The listing builds one solid part. Answer for the finished solid, in the listing's coordinates (mm). Give positions to 0.01 mm unless a question says otherwise; leave off trailing zeros. Order: outer loops, then holes, each group sorted by start corner. A loop starts at its lowest first (then second) coordinate and runs counter-clockwise, first axis right, second up. Notation, with made-up numbers: (86, 41) -> (131, 41) arc R9 ccw to (131, 47) -> close; hole circle Ø4 at (-14.5, 4). An arc over 180 degrees is marked (long way). Write item = value, one per line. Start each with the question number.
```python
from build123d import *

# Parameters (mm, degrees)
BOSS_EXTRUDE1_DEPTH = 5.08
SKETCH5_W           = 7.112
SKETCH5_H           = 7.112
SKETCH5_W_2         = 2.794
SKETCH5_H_2         = 43.434
CUT_EXTRUDE1_DEPTH  = 6.08


with BuildPart() as part:
    # Sketch1 → Boss-Extrude1 (new body)
    with BuildSketch(Plane.XY):
        Polygon((-4.120444444, 6.35), (53.34, 6.35), (53.34, -95.25), (16.22499019, -95.25), (-16.356614113, -78.274710363), (-26.416, -57.15), align=None)
    extrude(amount=BOSS_EXTRUDE1_DEPTH)

    # Sketch5 → Cut-Extrude1 (cut, through all)
    with BuildSketch(Plane(origin=(0, 0, 0), x_dir=(-1, 0, 0), z_dir=(0, 0, -1))):
        with Locations((-36.83, -17.78)):
            Rectangle(SKETCH5_W, SKETCH5_H)
        with Locations((-39.37, -45.72)):
            Rectangle(SKETCH5_W, SKETCH5_H)
        with Locations((-36.83, -27.94)):
            Rectangle(SKETCH5_W, SKETCH5_H)
        with Locations((-41.91, -64.77)):
            Rectangle(SKETCH5_W, SKETCH5_H)
        with Locations((-41.91, -83.82)):
            Rectangle(SKETCH5_W, SKETCH5_H)
        with Locations((-22.098, -17.78)):
            Rectangle(SKETCH5_W, SKETCH5_H)
        with Locations((-22.098, -27.94)):
            Rectangle(SKETCH5_W, SKETCH5_H)
        with Locations((-23.622, -45.72)):
            Rectangle(SKETCH5_W, SKETCH5_H)
        with Locations((-25.146, -64.77)):
            Rectangle(SKETCH5_W, SKETCH5_H)
        with Locations((-15.367, -26.543)):
            Rectangle(SKETCH5_W_2, SKETCH5_H_2)
        with Locations((-0.127, -26.543)):
            Rectangle(SKETCH5_W_2, SKETCH5_H_2)
    extrude(amount=-CUT_EXTRUDE1_DEPTH, mode=Mode.SUBTRACT)


solid = part.part
```
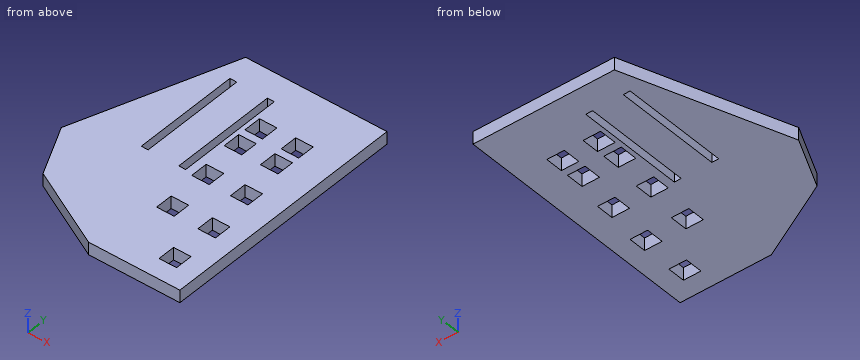
Item 1: Flat-ended cylindrical pins translate along their axes: pin 1 (3 mm diameter, centred on x = 14, y = -7, fed in from +Z); pin 2 (2.5 mm diameter, centred on y = -45, z = 2.5, fed in from -X); pin 3 (2.5 mm diameter, centred on y = -46, z = 1.5, fed in from -X); pin 4 (2.5 mm diameter, centred on y = -64.5, z = 2, fed in from -X). Find the tip coordinate at first contact, or state that the pin passes through.
Item 2: Consider L1, parallel to Y at x = 26.5, z = 1.5; L2, parallel to Y at x = 41, z = 4.6; L3, parallel to X at y = -16, z = 4.15. Determine where each line is inside the solid, lowest interval first. Write a range as from..to.
Item 3: A cutting plane is placed at B-B, the plane z = 2.65. Count the separate pieces of the cut face and the enclosed holes in it, plus the area to 3 significant figures.
Item 4: A cutting plane is placed at A-A, the plane y = -8. Write down the section's boundary in (x, z).
Item 5: A cutting plane is placed at C-C, the plane y = -71. Write down the section's boundary in (x, z).
Check values:
q1.pin_1 = 5.08
q1.pin_2 = -22.59
q1.pin_3 = -22.94
q1.pin_4 = -23.51
q2.L1 = -95.25..-68.33, -61.21..-49.28, -42.16..6.35
q2.L2 = -95.25..-87.38, -80.26..-68.33, -61.21..-49.28, -42.16..6.35
q2.L3 = -11.97..-1.27, 1.52..13.97, 16.76..18.54, 25.65..33.27, 40.39..53.34
q3.separate_pieces = 1
q3.enclosed_holes = 11
q3.area = 6,140 mm^2
q4.outline = (-9.16, 0) -> (-1.27, 0) -> (-1.27, 5.08) -> (-9.16, 5.08) -> close; (1.52, 0) -> (13.97, 0) -> (13.97, 5.08) -> (1.52, 5.08) -> close; (16.76, 0) -> (53.34, 0) -> (53.34, 5.08) -> (16.76, 5.08) -> close
q5.outline = (-19.82, 0) -> (53.34, 0) -> (53.34, 5.08) -> (-19.82, 5.08) -> close
